```python
from build123d import *

# Parameters (mm, degrees)
F0_W     = 18
F0_H     = 85
F1_DEPTH = 2
F2_W     = 2
F2_H     = 85
F3_DEPTH = 10
F4_W     = 85
F4_H     = 2
F5_DEPTH = 9
F6_W     = 85
F6_H     = 2
F7_DEPTH = 9


with BuildPart() as f1:
    # F0 (on Top) → F1 (new body)
    with BuildSketch(Plane.XY):
        with Locations((-9, 42.5)):
            Rectangle(F0_W, F0_H)
        with BuildLine():
            ThreePointArc((-12, 72), (-9, 81), (-6, 72))
            Line((-6, 72), (-6, 9))
            ThreePointArc((-6, 9), (-9, 6), (-12, 9))
            Line((-12, 9), (-12, 72))
        make_face(mode=Mode.SUBTRACT)
    extrude(amount=-F1_DEPTH)

    # F2 (on face) → F3 (join)
    with BuildSketch(Plane(origin=(0, 0, -2), x_dir=(1, 0, 0), z_dir=(0, 0, -1))):
        with Locations((-1, -42.5)):
            Rectangle(F2_W, F2_H)
        with Locations((-17, -42.5)):
            Rectangle(F2_W, F2_H)
    extrude(amount=F3_DEPTH)

    # F4 (on face) → F5 (join)
    with BuildSketch(Plane.YZ):
        with Locations((42.5, -11)):
            Rectangle(F4_W, F4_H)
    extrude(amount=F5_DEPTH)

    # F6 (on face) → F7 (join)
    with BuildSketch(Plane(origin=(-18, 0, 0), x_dir=(0, -1, 0), z_dir=(-1, 0, 0))):
        with Locations((-42.5, -11)):
            Rectangle(F6_W, F6_H)
    extrude(amount=F7_DEPTH)


solid = f1.part
```
Here's how the part is built. I have some questions about the finished solid (model axes, mm). A direction names the side the tool comes from. Give positions to 0.01 mm unless a question says otherwise; leave off trailing zeros. Loops run counter-clockwise (first coordinate to the right, second up) from the corner with the lowest first, then second, coordinate; pieces in that order, holes last. Notation, with made-up numbers: M -4.5,-22.75 L -0.5,-22.75 A7 ccw -0.5,-18.75 Z; hole C 27.5,-14.75 d1. An arc over 180 degrees is marked long. Put each result on its own line as item: value. Start each with the question number.
(1) I want a section at A-A on y = 76. Please give me the cut outline in (x, z), then the cut area to 3 significant figures.
(2) I want a section at D-D on y = 13.5. Please give me the cut outline in (x, z).
(3) I need wall thicknesses on line 1 along Y through (x, z) = (-9, -0.95); line 2 along X through (y, z) = (76, -0.65); line 3 along X through (y, z) = (19.5, -1.25). Which ranges of each line are inside material? Lowest first, please. Write a range as [from, to].
(4) If we mould it in two halves opening along X, with no side actions, what happens to faces 6 (the flat face through (-18, 42, -5)), 7 (the flat face through (-12, 40, -1)), 8 (the flat face through (-21, 43, -12))? For each: +X half, -X half, draft (parallel to the pull), parting line (faces both ways), or undercut.
(5) I want a section at C-C on x = -5. Please give me the cut outline in (y, z).
(6) Will these pins go through, and if not, where does the flat tip stop? pin 1 Ø0.6 at (y, z) = (51.5, -1) entering from -X; pin 2 Ø12 at (x, y) = (-6, 69) entering from +Z; pin 3 Ø1.5 at (x, y) = (-22, 55.5) entering from +Z; pin 4 Ø2 at (y, z) = (32, -1) entering from +X.
(7) For faces 1 (the flat face through (-22, 43, -10)), 2 (the flat face through (3, 42, -12)), 3 (the flat face through (0, 43, -5)), 4 (the flat face through (-16, 43, -7)), 5 (the cylindrical face through (-9, 6, -1)), which set-ups out of +Z, -Z, +X, -X, +Y, -Y let a thin tool reach every point of the face, with its end or its side?
(8) I want a section at B-B on z = -3.5. Please give me the cut outline in (x, y).
Answer block:
1. outline: M -27,-12 L -16,-12 L -16,-2 L -14,-2 L -14,0 L -18,0 L -18,-10 L -27,-10 Z; M -4,-2 L -2,-2 L -2,-12 L 9,-12 L 9,-10 L 0,-10 L 0,0 L -4,0 Z
1. area: 92.0 mm^2
2. outline: M -27,-12 L -16,-12 L -16,-2 L -12,-2 L -12,0 L -18,0 L -18,-10 L -27,-10 Z; M -6,-2 L -2,-2 L -2,-12 L 9,-12 L 9,-10 L 0,-10 L 0,0 L -6,0 Z
3. line 1: [0, 6], [81, 85]
3. line 2: [-18, -14], [-4, 0]
3. line 3: [-18, -12], [-6, 0]
4. face 6: -X half
4. face 7: undercut
4. face 8: draft
5. outline: M 0,-2 L 73,-2 L 73,0 L 0,0 Z; M 79,-2 L 85,-2 L 85,0 L 79,0 Z
6. pin 1: x = -18
6. pin 2: z = 0
6. pin 3: z = -10
6. pin 4: x = 0
7. face 1: +Z, -X, +Y, -Y
7. face 2: -Z, +X, -X, +Y, -Y
7. face 3: +Z, +X, +Y, -Y
7. face 4: -Z, +Y, -Y
7. face 5: +Z, -Z
8. outline: M -18,0 L -16,0 L -16,85 L -18,85 Z; M -2,0 L 0,0 L 0,85 L -2,85 Z
